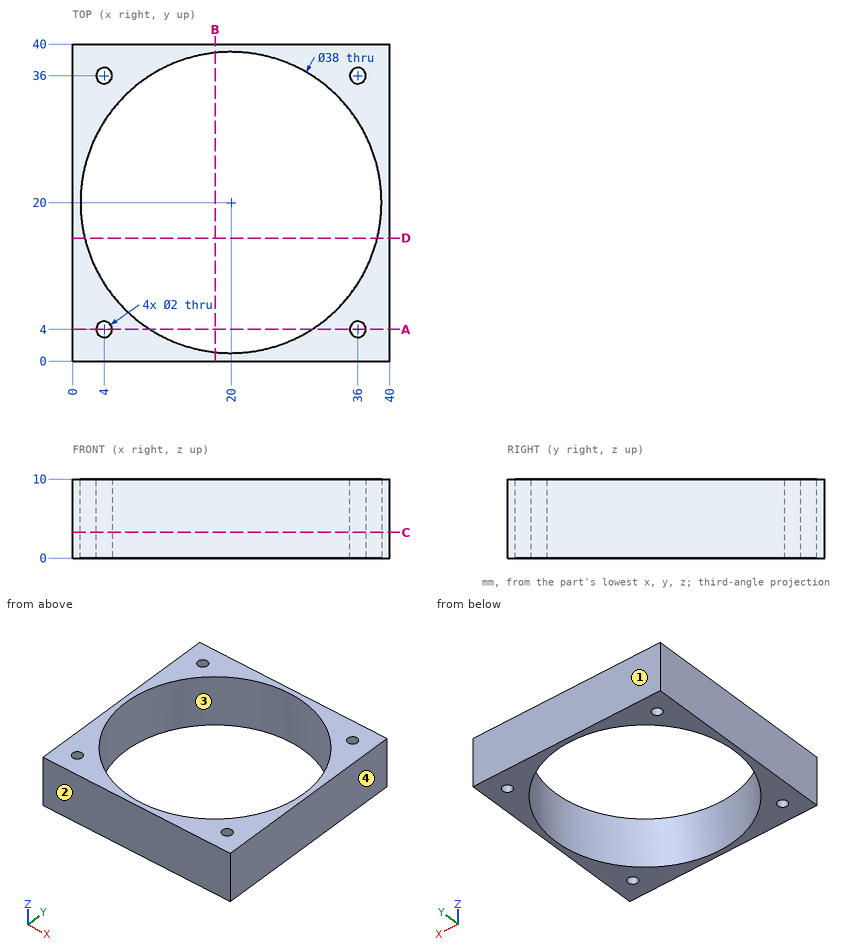
Job drawing, mm, ordinate dimensions from the low corner. One solid piece. Round coordinates to 2 decimals unless told otherwise and drop trailing zeros. Write each loop counter-clockwise with the first axis right and the second up, starting at its lowest first coordinate (ties: lowest second). Pieces come first, ordered by that corner, then holes.
1) Pin check, flat tips, straight feed: pin 1 (2 mm diameter, centred on y = 19, z = 4.5, fed in from -X); pin 2 (1.6 mm diameter, centred on x = 36, y = 36, fed in from +Z). Stop position of each tip, or through.
2) Band-saw the part on A-A, the plane y = 4. List the corners of the cut face in (x, z), and give its area (3 significant figures).
3) Band-saw the part on D-D, the plane y = 15.5. List the corners of the cut face in (x, z), and give its area (3 significant figures).
4) Band-saw the part on C-C, the plane z = 3.25. List the corners of the cut face in (x, y).
5) Mould opens along Y. For the marked faces 1, 2, 3 and 4 say: +Y half, -Y half, draft (parallel to the pull), parting line (faces both ways), or undercut.
6) Drill centre lines: probe 1 along Y at (x, z) = (4, 7.75); probe 2 along Y at (x, z) = (20, 9.75); probe 3 along X at (y, z) = (6, 7.5). Where is each one in solid material? Low to high.
7) Band-saw the part on B-B, the plane x = 18. List the corners of the cut face in (y, z).
Ans:
1. pin 1: stops at x = 0
1. pin 2: passes through
2. outline: (0, 0) - (3, 0) - (3, 10) - (0, 10) - close; (5, 0) - (9.75, 0) - (9.75, 10) - (5, 10) - close; (30.25, 0) - (35, 0) - (35, 10) - (30.25, 10) - close; (37, 0) - (40, 0) - (40, 10) - (37, 10) - close
2. area: 155 mm2
3. outline: (0, 0) - (1.54, 0) - (1.54, 10) - (0, 10) - close; (38.46, 0) - (40, 0) - (40, 10) - (38.46, 10) - close
3. area: 30.8 mm2
4. outline: (0, 0) - (40, 0) - (40, 40) - (0, 40) - close; hole circle Ø38 at (20, 20); hole circle Ø2 at (4, 4); hole circle Ø2 at (4, 36); hole circle Ø2 at (36, 4); hole circle Ø2 at (36, 36)
5. face 1: +Y half
5. face 2: -Y half
5. face 3: undercut
5. face 4: draft
6. probe 1: y = 0 to 3, 5 to 9.75, 30.25 to 35, 37 to 40
6. probe 2: y = 0 to 1, 39 to 40
6. probe 3: x = 0 to 7.15, 32.85 to 40
7. outline: (0, 0) - (1.11, 0) - (1.11, 10) - (0, 10) - close; (38.89, 0) - (40, 0) - (40, 10) - (38.89, 10) - close
